Check sheet for the drawn part. Datum: minimum x, y, z corner. Units: mm. Give positions to 0.01 mm unless a question says otherwise; leave off trailing zeros. Write each loop counter-clockwise with the first axis right and the second up, starting at its lowest first coordinate (ties: lowest second). Pieces come first, ordered by that corner, then holes. Notation, with made-up numbers: (25.25, 58) -> (69.25, 58) arc R29 ccw to (69.25, 96) -> close; hole circle Ø2 at (14, 59). An arc over 180 degrees is marked (long way). Answer as CSV lines item,"result". Start each with the question number.
1) Sectioned sample at B-B on y = 5.5. Record the cut outline in (x, z) (3 decimals).
2) Material ranges on L1, parallel to Y at x = 2.75, z = 1; L2, parallel to X at y = 10, z = 3.25; L3, parallel to Z at x = 5, y = 3.75, recorded low to high.
3) Gauge pin test, flat ends, axial feed: pin 1 Ø3 at (x, z) = (3, 2) entering from -Y; pin 2 Ø1 at (x, z) = (4, 2.5) entering from -Y; pin 3 Ø2 at (x, y) = (5, 11) entering from -Z. Record the tip position at first contact, or that the pin passes through.
4) Sectioned sample at D-D on x = 1.5. Record the cut outline in (y, z).
5) Sectioned sample at A-A on x = 4.5. Record the cut outline in (y, z), and give its area (3 significant figures).
6) Sectioned sample at C-C on z = 4.75. Record the cut outline in (x, y).
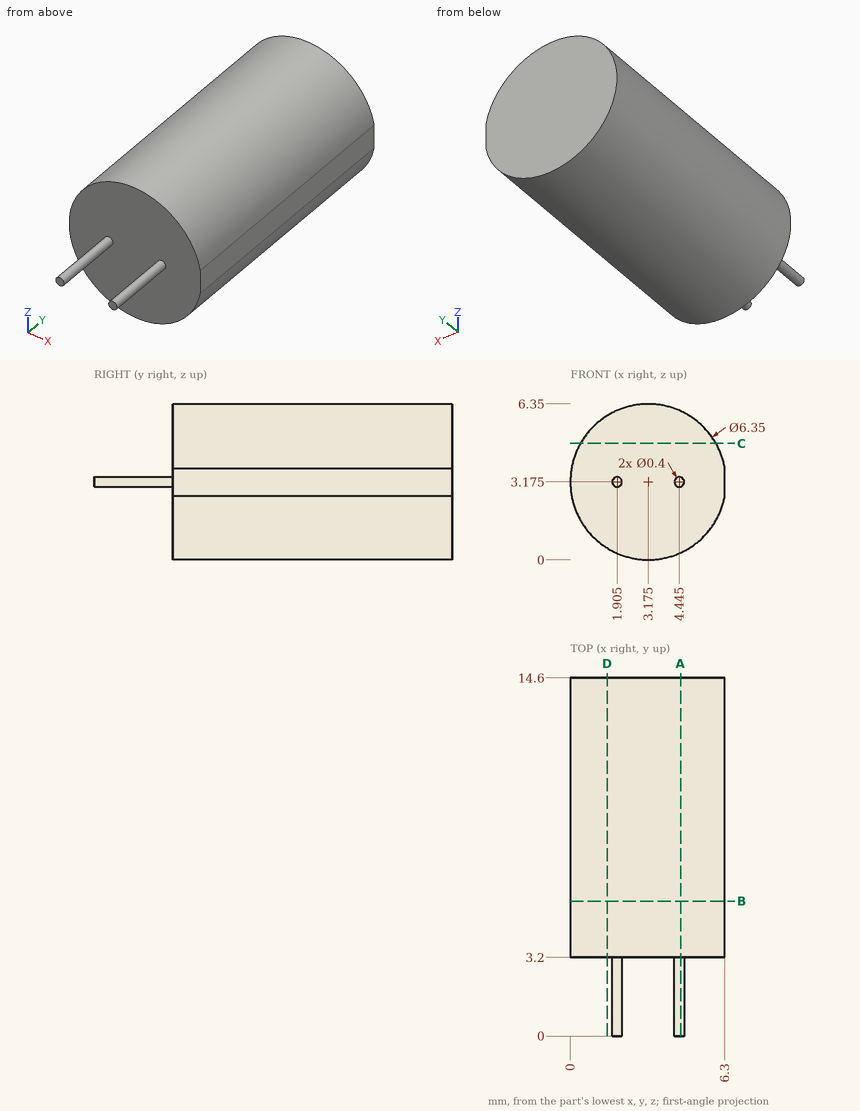
Ans:
1,outline,"(6.3, 2.614) -> (6.3, 3.736) arc R3.175 ccw (long way) to start"
2,L1,"y = 3.2 to 14.6"
2,L2,"x = 0 to 6.3"
2,L3,"z = 0.58 to 5.77"
3,pin 1,"stops at y = 0"
3,pin 2,"stops at y = 3.2"
3,pin 3,"stops at z = 0.11"
4,outline,"(3.2, 0.48) -> (14.6, 0.48) -> (14.6, 5.87) -> (3.2, 5.87) -> close"
5,outline,"(0, 2.98) -> (3.2, 2.98) -> (3.2, 0.29) -> (14.6, 0.29) -> (14.6, 6.06) -> (3.2, 6.06) -> (3.2, 3.37) -> (0, 3.37) -> close"
5,area,"67.0 mm²"
6,outline,"(0.42, 3.2) -> (5.93, 3.2) -> (5.93, 14.6) -> (0.42, 14.6) -> close"
